```python
from build123d import *

# Parameters (mm, degrees)
SKETCH_1_W               = 33
SKETCH_1_H               = 47
SKETCH_1_R               = 1.6
SKETCH_1_R_2             = 3.5
EXTRUDE_1_DEPTH          = 4
EXTRUDE_2_DEPTH          = 30
EXTRUDE_START            = -4
SKETCH_4_W               = 33
SKETCH_4_H               = 38
EXTRUDE_3_DEPTH          = 4
SKETCH_6_W               = 50
SKETCH_6_H               = 40
SKETCH_6_R               = 5.5
SKETCH_6_R_2             = 1.5
EXTRUDE_4_DEPTH          = 30
SKETCH_7_W               = 37.75
SKETCH_7_H               = 40
CUT_EXTRUDE_1_DEPTH      = 20
SKETCH_8_R               = 9.75
CUT_EXTRUDE_2_DEPTH      = 6.2
SKETCH_10_R              = 2.15
CUT_EXTRUDE_4_DEPTH      = 136.486392306
SKETCH_11_W              = 30
SKETCH_11_H              = 30
SKETCH_11_R              = 1.7
EXTRUDE_5_DEPTH          = 5
CUT_EXTRUDE_5_DEPTH      = 20
CHAMFER_1_SIZE           = 4
CHAMFER_2_SIZE           = 3
CHAMFER_3_SIZE           = 10
CUT_EXTRUDE_6_DEPTH      = 164.487193688
CUT_EXTRUDE_6_DEPTH_BACK = 30
SKETCH_13_W              = 132.923896649
SKETCH_13_H              = 188.96680941
SKETCH_14_W              = 30
SKETCH_14_H              = 20
SKETCH_14_R              = 2.15
EXTRUDE_6_DEPTH          = 0.5


with BuildPart() as part:
    # 草图1 → 凸台-拉伸1 (new body)
    with BuildSketch(Plane.XY):
        with Locations((16.5, 23.5)):
            Rectangle(SKETCH_1_W, SKETCH_1_H)
        with Locations((7.5, 40)):
            Circle(SKETCH_1_R, mode=Mode.SUBTRACT)
        with Locations((25.5, 40)):
            Circle(SKETCH_1_R, mode=Mode.SUBTRACT)
        with Locations((7.5, 7)):
            Circle(SKETCH_1_R, mode=Mode.SUBTRACT)
        with Locations((25.5, 7)):
            Circle(SKETCH_1_R, mode=Mode.SUBTRACT)
        with Locations((16.5, 31)):
            Circle(SKETCH_1_R_2, mode=Mode.SUBTRACT)
    extrude(amount=EXTRUDE_1_DEPTH)

    # 草图3 → 凸台-拉伸2 (add)
    with BuildSketch(Plane(origin=(0, 0, 0), x_dir=(-1, 0, 0), z_dir=(0, 0, -1))):
        Polygon((0, -38), (-33, -38), (-33, 47), (-39, 47), (-39, -63), (-26.75, -63), (-26.75, -43), (-6.25, -43), (-6.25, -63), (6, -63), (6, 47), (0, 47), align=None)
    extrude(amount=-EXTRUDE_2_DEPTH)

    # 草图4 → 凸台-拉伸3 (add)
    with BuildSketch(Plane(origin=(0, 0, 0), x_dir=(-1, 0, 0), z_dir=(0, 0, -1)).offset(EXTRUDE_START)):
        with Locations((-16.5, -19)):
            Rectangle(SKETCH_4_W, SKETCH_4_H)
    extrude(amount=EXTRUDE_3_DEPTH)

    # 草图6 → 凸台-拉伸4 (add, through all)
    with BuildSketch(Plane(origin=(0, 0, 0), x_dir=(-1, 0, 0), z_dir=(0, 0, -1))):
        with Locations((-51.75, -83)):
            Rectangle(SKETCH_6_W, SKETCH_6_H)
        with Locations((-56.75, -83)):
            Circle(SKETCH_6_R, mode=Mode.SUBTRACT)
        with Locations((-68.75, -95)):
            Circle(SKETCH_6_R_2, mode=Mode.SUBTRACT)
        with Locations((-68.75, -71)):
            Circle(SKETCH_6_R_2, mode=Mode.SUBTRACT)
        with Locations((-44.75, -95)):
            Circle(SKETCH_6_R_2, mode=Mode.SUBTRACT)
        with Locations((-44.75, -71)):
            Circle(SKETCH_6_R_2, mode=Mode.SUBTRACT)
    extrude(amount=-EXTRUDE_4_DEPTH)

    # 草图7 → 切除-拉伸1 (cut)
    with BuildSketch(Plane.XY.offset(30)):
        with Locations((57.875, -83)):
            Rectangle(SKETCH_7_W, SKETCH_7_H)
    extrude(amount=-CUT_EXTRUDE_1_DEPTH, mode=Mode.SUBTRACT)

    # 草图8 → 切除-拉伸2 (cut)
    with BuildSketch(Plane.XY.offset(10)):
        with Locations((56.75, -83)):
            Circle(SKETCH_8_R)
    extrude(amount=-CUT_EXTRUDE_2_DEPTH, mode=Mode.SUBTRACT)

    # 草图10 → 切除-拉伸4 (cut, through all)
    with BuildSketch(Plane.ZY.offset(6)):
        with Locations(Location((15, -53, 0), (0, 0, 270))):
            Circle(SKETCH_10_R)
    extrude(amount=-CUT_EXTRUDE_4_DEPTH, mode=Mode.SUBTRACT)

    # 草图11 → 凸台-拉伸5 (add)
    with BuildSketch(Plane.ZY.offset(-26.75)):
        with Locations((15, -118)):
            Rectangle(SKETCH_11_W, SKETCH_11_H)
        with Locations(Location((20, -118, 0), (0, 0, 270))):
            Circle(SKETCH_11_R, mode=Mode.SUBTRACT)
    extrude(amount=-EXTRUDE_5_DEPTH)

    # 草图12 → 切除-拉伸5 (cut)
    with BuildSketch(Plane.XY.offset(10)):
        Polygon((39, -103), (76.75, -103), (76.75, -63), (39, -63), (39, -66), (73.75, -66), (73.75, -100), (39, -100), align=None)
    extrude(amount=-CUT_EXTRUDE_5_DEPTH, mode=Mode.SUBTRACT)

    # 倒角1
    chamfer_1_edges = [part.edges().sort_by_distance(p)[0] for p in [
        (31.75, -103, 15),
        (-6, 47, 15),
        (-6, -63, 15),
        (39, 47, 15),
    ]]
    chamfer(chamfer_1_edges, length=CHAMFER_1_SIZE)

    # 倒角2
    chamfer_2_edges = [part.edges().sort_by_distance(p)[0] for p in [
        (39, -100, 5),
        (39, -66, 5),
    ]]
    chamfer(chamfer_2_edges, length=CHAMFER_2_SIZE - 0.0001)  # a hair under: the kernel refuses the full size
    chamfer_2_2_edges = [part.edges().sort_by_distance(p)[0] for p in [
        (73.75, -100, 5),
        (73.75, -66, 5),
    ]]
    chamfer(chamfer_2_2_edges, length=CHAMFER_2_SIZE)

    # 倒角3
    chamfer_3_edges = [part.edges().sort_by_distance(p)[0] for p in [
        (29.25, -133, 0),
    ]]
    chamfer(chamfer_3_edges, length=CHAMFER_3_SIZE)


with BuildPart() as body_2:
    # 镜向1: mirrored copy
    add(part.part.mirror(Plane(origin=(0, 0, 0), x_dir=(1, 0, 0), z_dir=(0, 0, -1))))

    # 草图14 → 凸台-拉伸6 (add)
    with BuildSketch(Plane(origin=(6.25, 0, 0), x_dir=(0, 0, -1), z_dir=(1, 0, 0))):
        with Locations((15, -53)):
            Rectangle(SKETCH_14_W, SKETCH_14_H)
        with Locations(Location((15, -53, 0), (0, 0, 270))):
            Circle(SKETCH_14_R, mode=Mode.SUBTRACT)
    extrude(amount=EXTRUDE_6_DEPTH)


with BuildPart() as part_1:
    add(part.part)

    # 草图13 → 切除-拉伸6 (cut, two sides: drawn at the far end of the back side and taken through both)
    with BuildSketch(Plane.XY.offset(30).offset(-CUT_EXTRUDE_6_DEPTH_BACK)):
        with Locations((27.793899124, -40.302373562)):
            Rectangle(SKETCH_13_W, SKETCH_13_H)
    extrude(amount=CUT_EXTRUDE_6_DEPTH + CUT_EXTRUDE_6_DEPTH_BACK, mode=Mode.SUBTRACT)


solid = body_2.part
```
The model under review builds one solid part; all positions refer to its coordinate system, in mm. A direction names the side the tool comes from. Give positions to 0.01 mm unless a question says otherwise; leave off trailing zeros. Write each loop counter-clockwise with the first axis right and the second up, starting at its lowest first coordinate (ties: lowest second). Pieces come first, ordered by that corner, then holes.
(1) Consider section D-D, the plane z = -6. Give the number of separate pieces and of enclosed holes in the cut face, and give its area (3 significant figures).
(2) Consider section B-B, the plane x = 16.5. Give the boundary of the cut face in (y, z).
(3) To check wall thickness, follow L1, parallel to Y at x = 25.5, z = -1; L2, parallel to X at y = -19.5, z = -15; L3, parallel to X at y = -46, z = -28. State the ranges of each line that lie inside material, in increasing order.
(4) Consider section A-A, the plane y = -53. Give the boundary of the cut face in (x, z).
(5) Consider section C-C, the plane y = -118. Give the boundary of the cut face in (x, z).
(6) Tool access review of faces 4 (the flat face through (29, -128, -5)), 5 (the cylindrical face through (44.945, -93.513, -4.93)), 6 (the flat face through (37, -103, -15)), 7 (the flat face through (6.75, -50.6, -14.8)), 8 (the flat face through (16, -38, -17)): name each direction out of +Z, -Z, +X, -X, +Y, -Y from which nothing blocks a thin tool from reaching the whole face with its end or side.
(7) For P1, Ø8, axis at x = 11, z = -14.5, coming from the +Y side; P2, Ø2, axis at y = -73, z = -18.5, coming from the -X side; P3, Ø4, axis at x = 44.75, y = -95, coming from the +Z side; P4, Ø9, axis at y = -52, z = -21.5, coming from the +X side, all flat-tipped, find the tip position at first contact; note any pin that passes through.
(8) The part is to be moulded in two halves that separate along Y. For faces 1 (the flat face through (2, -63, -15)), 2 (the flat face through (41, -65, -5)), 3 (the cylindrical face through (49.564, -76.41, -6.943)), say which applies: released by +Y, released by -Y, zero draft, split by the parting line, or undercut.
Returned:
1. separate pieces: 1
1. enclosed holes: 5
1. area: 3,200 mm2
2. outline: (-43, -30) - (-38, -30) - (-38, -4) - (27.5, -4) - (27.5, 0) - (-43, 0) - close; (34.5, -4) - (47, -4) - (47, 0) - (34.5, 0) - close
3. L1: y = -43 to 5.4, 8.6 to 38.4, 41.6 to 47
3. L2: x = -6 to 0, 33 to 39
3. L3: x = -6 to 6.75, 26.75 to 39
4. outline: (-6, -30) - (6.75, -30) - (6.75, -17.15) - (-6, -17.15) - close; (-6, -12.85) - (6.75, -12.85) - (6.75, 0) - (-6, 0) - close; (26.75, -30) - (39, -30) - (39, -17.15) - (26.75, -17.15) - close; (26.75, -12.85) - (39, -12.85) - (39, 0) - (26.75, 0) - close
5. outline: (26.75, -30) - (31.75, -30) - (31.75, -21.7) - (26.75, -21.7) - close; (26.75, -18.3) - (31.75, -18.3) - (31.75, 0) - (26.75, 0) - close
6. face 4: +Z, +X, -X, -Y
6. face 5: +Z, -Z
6. face 6: +Z, -Z, +X, -Y
6. face 7: +Z, -Z, -Y
6. face 8: -Z, +Y
7. P1: stops at y = -38
7. P2: stops at x = 26.75
7. P3: stops at z = 0
7. P4: stops at x = 39
8. face 1: released by -Y
8. face 2: released by +Y
8. face 3: undercut
